Geometry: final body of the model. Coordinates: model frame, mm. A direction names the side the tool comes from. Give positions to 0.01 mm unless a question says otherwise; leave off trailing zeros. Write each loop counter-clockwise with the first axis right and the second up, starting at its lowest first coordinate (ties: lowest second). Pieces come first, ordered by that corner, then holes. Notation, with made-up numbers: M 63,14.25 L 86,14.25 A29 cw 86,41.25 Z; hole C 68.5,-27 d4. An arc over 180 degrees is marked long. One line per question, with ' | ' between items.
from build123d import *

# Parameters (mm, degrees)
F1_DEPTH = 6
F3_D     = 6
F4_R     = 5


with BuildPart() as f1:
    # F0 (on Top) → F1 (new body)
    with BuildSketch(Plane.XY):
        with BuildLine():
            Line((7.5, -30), (7.5, 30))
            Line((7.5, 30), (-7.5, 30))
            Line((-7.5, 30), (-7.5, 11.83216))
            ThreePointArc((-7.5, 11.83216), (-3.5, 0), (-7.5, -11.83216))
            Line((-7.5, -11.83216), (-7.5, -30))
            Line((-7.5, -30), (7.5, -30))
        make_face()
    extrude(amount=F1_DEPTH)

    # F3 (through all)
    with Locations(Plane.XY.offset(6)):
        with Locations((0, 23.5), (0, -23.5)):
            Hole(F3_D / 2)

    # F4
    f4_edges = [f1.edges().sort_by_distance(p)[0] for p in [
        (7.5, 30, 3),
        (7.5, -30, 3),
        (-7.5, -11.83216, 3),
        (-7.5, 11.83216, 3),
    ]]
    fillet(f4_edges, radius=F4_R)


solid = f1.part
(1) Draft query along Y for faces 3 (the face through (0, 0, 0)), 4 (the face through (-7.3, -12.01, 3.04)), 5 (the face through (6.07, 28.5, 3.04)). Return one class per face: released by +Y, released by -Y, zero draft, split by the parting line, or undercut.
Working result:
face 3: zero draft | face 4: undercut | face 5: released by +Y
(2) First-contact query: P1, Ø1.5, axis at x = 4.5, z = 4, coming from the -Y side; P2, Ø5, axis at x = 0, y = 23.5, coming from the -Z side (3 decimals). Flat tips, straight axial feed; report the tip coordinate or a pass-through.
Working result:
P1: stops at y = -29.84 | P2: passes through
(3) Cut plane B-B, the plane x = 0. Return loops of the section in (y, z), then the cut area to 3 significant figures.
Working result:
outline: M -30,0 L -26.5,0 L -26.5,6 L -30,6 Z; M -20.5,0 L 20.5,0 L 20.5,6 L -20.5,6 Z; M 26.5,0 L 30,0 L 30,6 L 26.5,6 Z | area: 288 mm^2
(4) Set-up query: faces 1 (the face through (0, 0, 6)), 2 (the face through (-7.3, 12.01, 3.04)). Return all of +Z, -Z, +X, -X, +Y, -Y with unobstructed straight access to the full face (end or side cutting, diameter ignored); none if empty.
Working result:
face 1: +Z, +X, -X, +Y, -Y | face 2: +Z, -Z, -X
(5) Cut plane C-C, the plane z = 4.05. Return loops of the section in (x, y).
Working result:
outline: M -7.5,-30 L 2.5,-30 A5 ccw 7.5,-25 L 7.5,25 A5 ccw 2.5,30 L -7.5,30 L -7.5,13.42 A5 ccw -6.68,10.68 A19.5 cw -6.68,-10.68 A5 ccw -7.5,-13.42 Z; hole C 0,-23.5 d6; hole C 0,23.5 d6
(6) Cut plane A-A, the plane y = -23.5. Return loops of the section in (x, z).
Working result:
outline: M -7.5,0 L -3,0 L -3,6 L -7.5,6 Z; M 3,0 L 7.5,0 L 7.5,6 L 3,6 Z
(7) Cut plane D-D, the plane x = -2.5. Return loops of the section in (y, z).
Working result:
outline: M -30,0 L -25.16,0 L -25.16,6 L -30,6 Z; M -21.84,0 L 21.84,0 L 21.84,6 L -21.84,6 Z; M 25.16,0 L 30,0 L 30,6 L 25.16,6 Z
(8) Material intervals for L1, parallel to Y at x = 0, z = 2.3; L2, parallel to Y at x = -1.25, z = 2.8; L3, parallel to Y at x = -5, z = 4.85, sorted ascending. Write a range as [from, to].
Working result:
L1: y = [-30, -26.5], [-20.5, 20.5], [26.5, 30] | L2: y = [-30, -26.23], [-20.77, 20.77], [26.23, 30] | L3: y = [-30, -7.5], [7.5, 30]
